Geometry: final body of the model. Coordinates: model frame, mm. Coordinates: 2 decimals unless noted, no trailing zeros. Order: outer loops, then holes, each group sorted by start corner. A loop starts at its lowest first (then second) coordinate and runs counter-clockwise, first axis right, second up. Notation, with made-up numbers: (-14, 56) -> (26, 56) arc R34 ccw to (26, 95) -> close; hole circle Ø10 at (-20, 34). An arc over 180 degrees is marked (long way). Use one line per item in the form item = value.
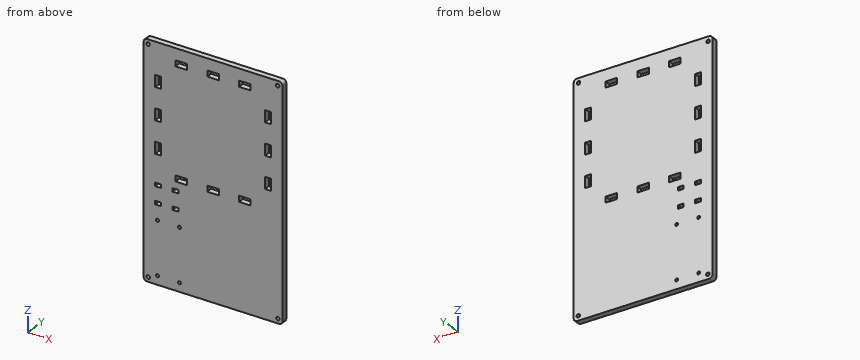
```python
from build123d import *

# Parameters (mm, degrees)
SKETCH1_W           = 120
SKETCH1_H           = 200
SKETCH1_R           = 1.5
SKETCH1_R_2         = 1.27
SKETCH1_W_2         = 5
SKETCH1_H_2         = 3
BOSS_EXTRUDE1_DEPTH = 5
CUT_EXTRUDE1_REACH  = 118.726
SKETCH4_W           = 5.1
SKETCH4_H           = 10
SKETCH4_W_2         = 10
SKETCH4_H_2         = 5.1
FILLET1_R           = 3


with BuildPart() as part:
    # Sketch1 → Boss-Extrude1 (new body)
    with BuildSketch(Plane(origin=(0, 0, 0), x_dir=(1, 0, 0), z_dir=(0, 1, 0))):
        Rectangle(SKETCH1_W, SKETCH1_H)
        with Locations(Location((-56, 96, 0), (0, 0, 270))):
            Circle(SKETCH1_R, mode=Mode.SUBTRACT)
        with Locations(Location((56, 96, 0), (0, 0, 270))):
            Circle(SKETCH1_R, mode=Mode.SUBTRACT)
        with Locations(Location((55.822222222, -96, 0), (0, 0, 270))):
            Circle(SKETCH1_R, mode=Mode.SUBTRACT)
        with Locations(Location((-56.177777778, -96, 0), (0, 0, 270))):
            Circle(SKETCH1_R, mode=Mode.SUBTRACT)
        with Locations(Location((-48.095, 92.46, 0), (0, 0, 270))):
            Circle(SKETCH1_R_2, mode=Mode.SUBTRACT)
        with Locations(Location((-29.045, 92.46, 0), (0, 0, 270))):
            Circle(SKETCH1_R_2, mode=Mode.SUBTRACT)
        with Locations(Location((-29.045, 46.74, 0), (0, 0, 270))):
            Circle(SKETCH1_R_2, mode=Mode.SUBTRACT)
        with Locations(Location((-48.095, 46.74, 0), (0, 0, 270))):
            Circle(SKETCH1_R_2, mode=Mode.SUBTRACT)
        with Locations((-32.5, 32.7)):
            Rectangle(SKETCH1_W_2, SKETCH1_H_2, mode=Mode.SUBTRACT)
        with Locations((-47.5, 32.7)):
            Rectangle(SKETCH1_W_2, SKETCH1_H_2, mode=Mode.SUBTRACT)
        with Locations((-32.5, 17.7)):
            Rectangle(SKETCH1_W_2, SKETCH1_H_2, mode=Mode.SUBTRACT)
        with Locations((-47.5, 17.7)):
            Rectangle(SKETCH1_W_2, SKETCH1_H_2, mode=Mode.SUBTRACT)
    extrude(amount=BOSS_EXTRUDE1_DEPTH)

    # Sketch4 → Cut-Extrude1 (cut, up to next)
    with BuildSketch(Plane(origin=(0, 5, 0), x_dir=(1, 0, 0), z_dir=(0, 1, 0)), mode=Mode.PRIVATE) as cut_extrude1_sk1:
        with Locations((-47.45, -12.5)):
            Rectangle(SKETCH4_W, SKETCH4_H)
    cut_extrude1_tool1 = extrude(cut_extrude1_sk1.sketch, amount=-CUT_EXTRUDE1_REACH, mode=Mode.PRIVATE) & part.part
    # Sketch4 → Cut-Extrude1 (cut, up to next)
    with BuildSketch(Plane(origin=(0, 5, 0), x_dir=(1, 0, 0), z_dir=(0, 1, 0)), mode=Mode.PRIVATE) as cut_extrude1_sk2:
        with Locations((-47.45, -67.5)):
            Rectangle(SKETCH4_W, SKETCH4_H)
    cut_extrude1_tool2 = extrude(cut_extrude1_sk2.sketch, amount=-CUT_EXTRUDE1_REACH, mode=Mode.PRIVATE) & part.part
    # Sketch4 → Cut-Extrude1 (cut, up to next)
    with BuildSketch(Plane(origin=(0, 5, 0), x_dir=(1, 0, 0), z_dir=(0, 1, 0)), mode=Mode.PRIVATE) as cut_extrude1_sk3:
        with Locations((-47.45, -40)):
            Rectangle(SKETCH4_W, SKETCH4_H)
    cut_extrude1_tool3 = extrude(cut_extrude1_sk3.sketch, amount=-CUT_EXTRUDE1_REACH, mode=Mode.PRIVATE) & part.part
    # Sketch4 → Cut-Extrude1 (cut, up to next)
    with BuildSketch(Plane(origin=(0, 5, 0), x_dir=(1, 0, 0), z_dir=(0, 1, 0)), mode=Mode.PRIVATE) as cut_extrude1_sk4:
        with Locations((-27.5, 7.45)):
            Rectangle(SKETCH4_W_2, SKETCH4_H_2)
    cut_extrude1_tool4 = extrude(cut_extrude1_sk4.sketch, amount=-CUT_EXTRUDE1_REACH, mode=Mode.PRIVATE) & part.part
    # Sketch4 → Cut-Extrude1 (cut, up to next)
    with BuildSketch(Plane(origin=(0, 5, 0), x_dir=(1, 0, 0), z_dir=(0, 1, 0)), mode=Mode.PRIVATE) as cut_extrude1_sk5:
        with Locations((0, 7.45)):
            Rectangle(SKETCH4_W_2, SKETCH4_H_2)
    cut_extrude1_tool5 = extrude(cut_extrude1_sk5.sketch, amount=-CUT_EXTRUDE1_REACH, mode=Mode.PRIVATE) & part.part
    # Sketch4 → Cut-Extrude1 (cut, up to next)
    with BuildSketch(Plane(origin=(0, 5, 0), x_dir=(1, 0, 0), z_dir=(0, 1, 0)), mode=Mode.PRIVATE) as cut_extrude1_sk6:
        with Locations((27.5, 7.45)):
            Rectangle(SKETCH4_W_2, SKETCH4_H_2)
    cut_extrude1_tool6 = extrude(cut_extrude1_sk6.sketch, amount=-CUT_EXTRUDE1_REACH, mode=Mode.PRIVATE) & part.part
    # Sketch4 → Cut-Extrude1 (cut, up to next)
    with BuildSketch(Plane(origin=(0, 5, 0), x_dir=(1, 0, 0), z_dir=(0, 1, 0)), mode=Mode.PRIVATE) as cut_extrude1_sk7:
        with Locations((47.45, -12.5)):
            Rectangle(SKETCH4_W, SKETCH4_H)
    cut_extrude1_tool7 = extrude(cut_extrude1_sk7.sketch, amount=-CUT_EXTRUDE1_REACH, mode=Mode.PRIVATE) & part.part
    # Sketch4 → Cut-Extrude1 (cut, up to next)
    with BuildSketch(Plane(origin=(0, 5, 0), x_dir=(1, 0, 0), z_dir=(0, 1, 0)), mode=Mode.PRIVATE) as cut_extrude1_sk8:
        with Locations((47.45, -40)):
            Rectangle(SKETCH4_W, SKETCH4_H)
    cut_extrude1_tool8 = extrude(cut_extrude1_sk8.sketch, amount=-CUT_EXTRUDE1_REACH, mode=Mode.PRIVATE) & part.part
    # Sketch4 → Cut-Extrude1 (cut, up to next)
    with BuildSketch(Plane(origin=(0, 5, 0), x_dir=(1, 0, 0), z_dir=(0, 1, 0)), mode=Mode.PRIVATE) as cut_extrude1_sk9:
        with Locations((47.45, -67.5)):
            Rectangle(SKETCH4_W, SKETCH4_H)
    cut_extrude1_tool9 = extrude(cut_extrude1_sk9.sketch, amount=-CUT_EXTRUDE1_REACH, mode=Mode.PRIVATE) & part.part
    # Sketch4 → Cut-Extrude1 (cut, up to next)
    with BuildSketch(Plane(origin=(0, 5, 0), x_dir=(1, 0, 0), z_dir=(0, 1, 0)), mode=Mode.PRIVATE) as cut_extrude1_sk10:
        with Locations((0, -87.45)):
            Rectangle(SKETCH4_W_2, SKETCH4_H_2)
    cut_extrude1_tool10 = extrude(cut_extrude1_sk10.sketch, amount=-CUT_EXTRUDE1_REACH, mode=Mode.PRIVATE) & part.part
    # Sketch4 → Cut-Extrude1 (cut, up to next)
    with BuildSketch(Plane(origin=(0, 5, 0), x_dir=(1, 0, 0), z_dir=(0, 1, 0)), mode=Mode.PRIVATE) as cut_extrude1_sk11:
        with Locations((-27.5, -87.45)):
            Rectangle(SKETCH4_W_2, SKETCH4_H_2)
    cut_extrude1_tool11 = extrude(cut_extrude1_sk11.sketch, amount=-CUT_EXTRUDE1_REACH, mode=Mode.PRIVATE) & part.part
    # Sketch4 → Cut-Extrude1 (cut, up to next)
    with BuildSketch(Plane(origin=(0, 5, 0), x_dir=(1, 0, 0), z_dir=(0, 1, 0)), mode=Mode.PRIVATE) as cut_extrude1_sk12:
        with Locations((27.5, -87.45)):
            Rectangle(SKETCH4_W_2, SKETCH4_H_2)
    cut_extrude1_tool12 = extrude(cut_extrude1_sk12.sketch, amount=-CUT_EXTRUDE1_REACH, mode=Mode.PRIVATE) & part.part
    add(cut_extrude1_tool1.solids().sort_by_distance((-47.45, 5, 12.5))[0], mode=Mode.SUBTRACT)
    add(cut_extrude1_tool2.solids().sort_by_distance((-47.45, 5, 67.5))[0], mode=Mode.SUBTRACT)
    add(cut_extrude1_tool3.solids().sort_by_distance((-47.45, 5, 40))[0], mode=Mode.SUBTRACT)
    add(cut_extrude1_tool4.solids().sort_by_distance((-27.5, 5, -7.45))[0], mode=Mode.SUBTRACT)
    add(cut_extrude1_tool5.solids().sort_by_distance((0, 5, -7.45))[0], mode=Mode.SUBTRACT)
    add(cut_extrude1_tool6.solids().sort_by_distance((27.5, 5, -7.45))[0], mode=Mode.SUBTRACT)
    add(cut_extrude1_tool7.solids().sort_by_distance((47.45, 5, 12.5))[0], mode=Mode.SUBTRACT)
    add(cut_extrude1_tool8.solids().sort_by_distance((47.45, 5, 40))[0], mode=Mode.SUBTRACT)
    add(cut_extrude1_tool9.solids().sort_by_distance((47.45, 5, 67.5))[0], mode=Mode.SUBTRACT)
    add(cut_extrude1_tool10.solids().sort_by_distance((0, 5, 87.45))[0], mode=Mode.SUBTRACT)
    add(cut_extrude1_tool11.solids().sort_by_distance((-27.5, 5, 87.45))[0], mode=Mode.SUBTRACT)
    add(cut_extrude1_tool12.solids().sort_by_distance((27.5, 5, 87.45))[0], mode=Mode.SUBTRACT)

    # Fillet1
    fillet1_edges = [part.edges().sort_by_distance(p)[0] for p in [
        (-60, 2.5, 100),
        (-60, 2.5, -100),
        (60, 2.5, -100),
        (60, 2.5, 100),
    ]]
    fillet(fillet1_edges, radius=FILLET1_R)


solid = part.part
```
1) Contact query for a flat-ended pin moving along its axis: P1, Ø1.5, axis at x = -48.095, z = -46.74, coming from the -Y side. Output: stop coordinate, or through.
Results found:
P1 = through
2) Material intervals for probe 1 along X at (y, z) = (1.4, 96); probe 2 along X at (y, z) = (4.35, -18.5); probe 3 along Z at (x, y) = (49, 4), sorted ascending. Write a range as from..to.
Results found:
probe_1 = -60..-57.68, -54.68..54.32, 57.32..60
probe_2 = -60..-50, -45..-35, -30..60
probe_3 = -100..7.5, 17.5..35, 45..62.5, 72.5..100
3) Section A-A, the plane z = 38.5. Output: boundary loops of the cut face in (x, y), and give its area (3 significant figures).
Results found:
outline = (-60, 0) -> (-50, 0) -> (-50, 5) -> (-60, 5) -> close; (-44.9, 0) -> (44.9, 0) -> (44.9, 5) -> (-44.9, 5) -> close; (50, 0) -> (60, 0) -> (60, 5) -> (50, 5) -> close
area = 549 mm2
4) Section B-B, the plane y = 4. Give the number of separate pieces and of enclosed holes in the cut face, and give its area (3 significant figures).
Results found:
separate_pieces = 1
enclosed_holes = 24
area = 23,300 mm2
